```python
from build123d import *

# Parameters (mm, degrees)
ESQUISSE1_W                = 28.3
ESQUISSE1_H                = 28.3
ESQUISSE1_W_2              = 20.3
ESQUISSE1_H_2              = 20.3
ESQUISSE1_W_3              = 4
ESQUISSE1_H_3              = 2
BOSS_EXTRU_1_DEPTH         = 20
BOSS_EXTRU_7_DEPTH         = 20
ESQUISSE2_W                = 8.5
ESQUISSE2_H                = 20
ESQUISSE2_R                = 1.7
BOSS_EXTRU_2_DEPTH         = 2
ESQUISSE2_3_W              = 8.5
ESQUISSE2_3_H              = 20
BOSS_EXTRU_3_DEPTH         = 3
ESQUISSE3_W                = 8.5
ESQUISSE3_H                = 20
ESQUISSE3_R                = 1.7
BOSS_EXTRU_4_DEPTH         = 2
ESQUISSE5_W                = 8.5
ESQUISSE5_H                = 20
ESQUISSE5_R                = 3
BOSS_EXTRU_5_DEPTH         = 2
BOSS_EXTRU_6_DEPTH         = 20
BOSS_EXTRU_6_DEPTH_BACK    = 20
ESQUISSE6_W                = 28.3
ESQUISSE6_H                = 28.3
ESQUISSE6_W_2              = 15.3
ESQUISSE6_H_2              = 15.3
BOSS_EXTRU_12_REACH        = 59.663
ESQUISSE20_W               = 28.3
ESQUISSE20_H               = 28.3
ENL_V_MAT_EXTRU_1_REACH    = 81.469
ESQUISSE7_W                = 6.5
ESQUISSE7_H                = 2
ENL_V_MAT_EXTRU_2_REACH    = 82.765
ESQUISSE8_W                = 14.15
ESQUISSE8_H                = 2
ESQUISSE9_W                = 8.5
ESQUISSE9_H                = 40
BOSS_EXTRU_8_DEPTH         = 5
ESQUISSE9_4_R              = 1.7
BOSS_EXTRU_9_DEPTH         = 2
ESQUISSE10_W               = 8.5
ESQUISSE10_H               = 40
ESQUISSE10_R               = 1.7
BOSS_EXTRU_10_DEPTH        = 2
ESQUISSE11_W               = 8.5
ESQUISSE11_H               = 40
ESQUISSE11_R               = 3
BOSS_EXTRU_11_DEPTH        = 2
NERVURE4_REACH             = 81.469
ESQUISSE14_WALL_W          = 172.71321229
ESQUISSE14_WALL_H          = 5
NERVURE10_REACH            = 81.469
ESQUISSE16_WALL_W          = 173.426178518
ESQUISSE16_WALL_H          = 5
R_P_TITION_LIN_AIRE1_COUNT = 3
R_P_TITION_LIN_AIRE1_PITCH = 17.5
NERVURE11_REACH            = 93.316
ESQUISSE17_WALL_W          = 197.121376998
ESQUISSE17_WALL_H          = 5
NERVURE17_REACH            = 75.701
ESQUISSE19_WALL_W          = 161.177827304
ESQUISSE19_WALL_H          = 5
R_P_TITION_LIN_AIRE2_COUNT = 2
R_P_TITION_LIN_AIRE2_PITCH = 15
R_P_TITION_LIN_AIRE3_COUNT = 2
R_P_TITION_LIN_AIRE3_PITCH = 15
ENL_V_MAT_EXTRU_3_REACH    = 75.701
ESQUISSE21_W               = 4
ESQUISSE21_H               = 2.012776607


with BuildPart() as part:
    # Esquisse1 → Boss.-Extru.1 (new body)
    # profile 1 of 2: a face of its own
    with BuildSketch(Plane.XY):
        Rectangle(ESQUISSE1_W, ESQUISSE1_H)
        Rectangle(ESQUISSE1_W_2, ESQUISSE1_H_2, mode=Mode.SUBTRACT)
    # profile 2 of 2: a face of its own
    with BuildSketch(Plane.XY):
        with Locations((12.15, -1)):
            Rectangle(ESQUISSE1_W_3, ESQUISSE1_H_3)
    extrude(amount=BOSS_EXTRU_1_DEPTH)

    # Esquisse1<3> → Boss.-Extru.7 (add)
    with BuildSketch(Plane.XY):
        Polygon((14.15, 14.15), (-14.15, 14.15), (-14.15, -14.15), (14.15, -14.15), (14.15, -2), (10.15, -2), (10.15, -10.15), (-10.15, -10.15), (-10.15, 10.15), (10.15, 10.15), (10.15, 0), (14.15, 0), align=None)
    extrude(amount=-BOSS_EXTRU_7_DEPTH)

    # Esquisse2 → Boss.-Extru.2 (add)
    with BuildSketch(Plane(origin=(0, 2, 0), x_dir=(-1, 0, 0), z_dir=(0, -1, 0))):
        with Locations((-18.4, 10)):
            Rectangle(ESQUISSE2_W, ESQUISSE2_H)
        with Locations(Location((-18.4, 10, 0), (0, 0, 180))):
            Circle(ESQUISSE2_R, mode=Mode.SUBTRACT)
    extrude(amount=BOSS_EXTRU_2_DEPTH)

    # Esquisse2<3> → Boss.-Extru.3 (add)
    with BuildSketch(Plane(origin=(0, 2, 0), x_dir=(-1, 0, 0), z_dir=(0, -1, 0))):
        with Locations((-18.4, 10)):
            Rectangle(ESQUISSE2_3_W, ESQUISSE2_3_H)
        Polygon((-15.65, 11.58771324), (-15.65, 8.41228676), (-18.4, 6.824573519), (-21.15, 8.41228676), (-21.15, 11.58771324), (-18.4, 13.175426481), align=None, mode=Mode.SUBTRACT)
    extrude(amount=-BOSS_EXTRU_3_DEPTH)

    # Esquisse3 → Boss.-Extru.4 (add)
    with BuildSketch(Plane(origin=(0, -2, 0), x_dir=(1, 0, 0), z_dir=(0, 1, 0))):
        with Locations((18.4, 10)):
            Rectangle(ESQUISSE3_W, ESQUISSE3_H)
        with Locations((18.4, 10)):
            Circle(ESQUISSE3_R, mode=Mode.SUBTRACT)
    extrude(amount=-BOSS_EXTRU_4_DEPTH)

    # Esquisse5 → Boss.-Extru.5 (add)
    with BuildSketch(Plane.XZ.offset(4)):
        with Locations((18.4, -10)):
            Rectangle(ESQUISSE5_W, ESQUISSE5_H)
        with Locations((18.4, -10)):
            Circle(ESQUISSE5_R, mode=Mode.SUBTRACT)
    extrude(amount=BOSS_EXTRU_5_DEPTH)


with BuildPart() as body_2:
    # Esquisse6 → Boss.-Extru.6 (new, two sides: drawn at the far end of the back side and taken through both)
    with BuildSketch(Plane(origin=(0, -11.88296393, 7.558102729), x_dir=(-1, 0, 0), z_dir=(0, -0.8660254037844382, 0.5000000000000011)).offset(-BOSS_EXTRU_6_DEPTH_BACK)):
        with Locations((0, -37.941481073)):
            Rectangle(ESQUISSE6_W, ESQUISSE6_H)
        with Locations((0, -37.941481073)):
            Rectangle(ESQUISSE6_W_2, ESQUISSE6_H_2, mode=Mode.SUBTRACT)
    extrude(amount=BOSS_EXTRU_6_DEPTH + BOSS_EXTRU_6_DEPTH_BACK)

    # Esquisse20 → Boss.-Extru.12 (add, up to next)
    with BuildSketch(Plane.XY.offset(20), mode=Mode.PRIVATE) as boss_extru_12_sk1:
        Rectangle(ESQUISSE20_W, ESQUISSE20_H)
    boss_extru_12_tool1 = extrude(boss_extru_12_sk1.sketch, amount=BOSS_EXTRU_12_REACH, mode=Mode.PRIVATE) - body_2.part

    add(part.part)  # Boss.-Extru.12 merges part
    add(boss_extru_12_tool1.solids().sort_by_distance((0, 0, 20))[0])

    # Esquisse7 → Enlèv. mat.-Extru.1 (cut, up to next)
    with BuildSketch(Plane(origin=(0, -29.505485507, 17.035), x_dir=(1, 0, 0), z_dir=(0, -0.866025403784438, 0.5000000000000011)), mode=Mode.PRIVATE) as enl_v_mat_extru_1_sk1:
        with Locations((10.9, 39.545508076)):
            Rectangle(ESQUISSE7_W, ESQUISSE7_H)
    enl_v_mat_extru_1_tool1 = extrude(enl_v_mat_extru_1_sk1.sketch, amount=-ENL_V_MAT_EXTRU_1_REACH, mode=Mode.PRIVATE) & body_2.part
    add(enl_v_mat_extru_1_tool1.solids().sort_by_distance((10.9, -9.732731, 51.282415))[0], mode=Mode.SUBTRACT)

    # Esquisse8 → Enlèv. mat.-Extru.2 (cut, up to next)
    with BuildSketch(Plane.XZ.offset(14.15), mode=Mode.PRIVATE) as enl_v_mat_extru_2_sk1:
        with Locations((7.075, 9.169506309)):
            Rectangle(ESQUISSE8_W, ESQUISSE8_H)
    enl_v_mat_extru_2_tool1 = extrude(enl_v_mat_extru_2_sk1.sketch, amount=-ENL_V_MAT_EXTRU_2_REACH, mode=Mode.PRIVATE) & body_2.part
    add(enl_v_mat_extru_2_tool1.solids().sort_by_distance((7.075, -14.15, 9.169506))[0], mode=Mode.SUBTRACT)

    # Esquisse9 → Boss.-Extru.8 (add)
    with BuildSketch(Plane(origin=(0, 19.272754038, 33.381389195), x_dir=(1, 0, 0), z_dir=(0, 0.5000000000000011, 0.866025403784438))):
        with Locations((18.4, -14.07)):
            Rectangle(ESQUISSE9_W, ESQUISSE9_H)
        Polygon((18.4, -7.245426481), (21.15, -5.65771324), (21.15, -2.48228676), (18.4, -0.894573519), (15.65, -2.48228676), (15.65, -5.65771324), align=None, mode=Mode.SUBTRACT)
        Polygon((18.4, -20.894573519), (21.15, -22.48228676), (21.15, -25.65771324), (18.4, -27.245426481), (15.65, -25.65771324), (15.65, -22.48228676), align=None, mode=Mode.SUBTRACT)
    extrude(amount=-BOSS_EXTRU_8_DEPTH)

    # Esquisse9<4> → Boss.-Extru.9 (add)
    # profile 1 of 2: a face of its own
    with BuildSketch(Plane(origin=(0, 19.272754038, 33.381389195), x_dir=(1, 0, 0), z_dir=(0, 0.5000000000000011, 0.866025403784438))):
        Polygon((15.65, -5.65771324), (18.4, -7.245426481), (21.15, -5.65771324), (21.15, -2.48228676), (18.4, -0.894573519), (15.65, -2.48228676), align=None)
        with Locations(Location((18.4, -4.07, 0), (0, 0, 270))):
            Circle(ESQUISSE9_4_R, mode=Mode.SUBTRACT)
    # profile 2 of 2: a face of its own
    with BuildSketch(Plane(origin=(0, 19.272754038, 33.381389195), x_dir=(1, 0, 0), z_dir=(0, 0.5000000000000011, 0.866025403784438))):
        Polygon((21.15, -22.48228676), (21.15, -25.65771324), (18.4, -27.245426481), (15.65, -25.65771324), (15.65, -22.48228676), (18.4, -20.894573519), align=None)
        with Locations(Location((18.4, -24.07, 0), (0, 0, 270))):
            Circle(ESQUISSE9_4_R, mode=Mode.SUBTRACT)
    extrude(amount=-BOSS_EXTRU_9_DEPTH)

    # Esquisse10 → Boss.-Extru.10 (add)
    with BuildSketch(Plane(origin=(0, 20.272754038, 35.113440003), x_dir=(-1, 0, 0), z_dir=(0, -0.5000000000000011, -0.866025403784438))):
        with Locations((-18.4, -14.07)):
            Rectangle(ESQUISSE10_W, ESQUISSE10_H)
        with Locations(Location((-18.4, -24.07, 0), (0, 0, 270))):
            Circle(ESQUISSE10_R, mode=Mode.SUBTRACT)
        with Locations(Location((-18.4, -4.07, 0), (0, 0, 270))):
            Circle(ESQUISSE10_R, mode=Mode.SUBTRACT)
    extrude(amount=-BOSS_EXTRU_10_DEPTH)

    # Esquisse11 → Boss.-Extru.11 (add)
    with BuildSketch(Plane(origin=(0, 21.272754038, 36.84549081), x_dir=(1, 0, 0), z_dir=(0, 0.5000000000000011, 0.866025403784438))):
        with Locations((18.4, -14.07)):
            Rectangle(ESQUISSE11_W, ESQUISSE11_H)
        with Locations(Location((18.4, -4.07, 0), (0, 0, 270))):
            Circle(ESQUISSE11_R, mode=Mode.SUBTRACT)
        with Locations(Location((18.4, -24.07, 0), (0, 0, 270))):
            Circle(ESQUISSE11_R, mode=Mode.SUBTRACT)
    extrude(amount=BOSS_EXTRU_11_DEPTH)

    # Esquisse14 wall → Nervure4 (add, up to next)
    with BuildSketch(Plane(origin=(18.4, -5.195231469, 59.141595139), x_dir=(0.721811427089, -0.346044890046, -0.599367331272), z_dir=(0.692089780103, 0.360905713545, 0.625107032601)), mode=Mode.PRIVATE) as nervure4_sk1:
        with Locations((0, 2.5)):
            Rectangle(ESQUISSE14_WALL_W, ESQUISSE14_WALL_H)
    nervure4_tool1 = extrude(nervure4_sk1.sketch, amount=-NERVURE4_REACH, mode=Mode.PRIVATE) - body_2.part
    nervure4 = nervure4_tool1.solids().sort_by_distance((18.4, -5.195231469, 59.141595139))[0]
    add(nervure4)

    # Esquisse16 wall → Nervure10 (add, up to next)
    with BuildSketch(Plane(origin=(18.4, -15.020231469, 42.124195954), x_dir=(-0.680604645529, -0.366325441564, -0.634494276844), z_dir=(0.732650883085, -0.340302322764, -0.589420912962)), mode=Mode.PRIVATE) as nervure10_sk1:
        with Locations((0, 2.5)):
            Rectangle(ESQUISSE16_WALL_W, ESQUISSE16_WALL_H)
    nervure10_tool1 = extrude(nervure10_sk1.sketch, amount=-NERVURE10_REACH, mode=Mode.PRIVATE) - body_2.part
    nervure10 = nervure10_tool1.solids().sort_by_distance((18.4, -15.020231469, 42.124195954))[0]
    add(nervure10)

    # Répétition linéaire1: Nervure4, Nervure10 ×3
    with Locations(*[Vector(0, 0.8660254037844382, -0.500000000000001) * (i * R_P_TITION_LIN_AIRE1_PITCH) for i in range(1, R_P_TITION_LIN_AIRE1_COUNT)]):
        add(nervure4)
        add(nervure10)

    # Esquisse17 wall → Nervure11 (add, up to next)
    with BuildSketch(Plane(origin=(18.4, 9.575, -20), x_dir=(-0.680604645507, 0.732650883105, 0), z_dir=(0.732650883105, 0.680604645507, 0)), mode=Mode.PRIVATE) as nervure11_sk1:
        with Locations((0, 2.5)):
            Rectangle(ESQUISSE17_WALL_W, ESQUISSE17_WALL_H)
    nervure11_tool1 = extrude(nervure11_sk1.sketch, amount=-NERVURE11_REACH, mode=Mode.PRIVATE) - body_2.part
    nervure11 = nervure11_tool1.solids().sort_by_distance((18.4, 9.575, -20))[0]
    add(nervure11)

    # Esquisse19 wall → Nervure17 (add, up to next)
    with BuildSketch(Plane(origin=(18.4, -10.075, 0), x_dir=(-0.721811427095, -0.692089780097, 0), z_dir=(0.692089780097, -0.721811427095, 0)), mode=Mode.PRIVATE) as nervure17_sk1:
        with Locations((0, 2.5)):
            Rectangle(ESQUISSE19_WALL_W, ESQUISSE19_WALL_H)
    nervure17_tool1 = extrude(nervure17_sk1.sketch, amount=-NERVURE17_REACH, mode=Mode.PRIVATE) - body_2.part
    nervure17 = nervure17_tool1.solids().sort_by_distance((18.4, -10.075, 0))[0]
    add(nervure17)

    # Répétition linéaire2: Nervure17 ×2
    with Locations(*[(0, 0, -i * R_P_TITION_LIN_AIRE2_PITCH) for i in range(1, R_P_TITION_LIN_AIRE2_COUNT)]):
        add(nervure17)

    # Répétition linéaire3: Nervure11 ×2
    with Locations(*[(0, 0, i * R_P_TITION_LIN_AIRE3_PITCH) for i in range(1, R_P_TITION_LIN_AIRE3_COUNT)]):
        add(nervure11)

    # Esquisse21 → Enlèv. mat.-Extru.3 (cut, up to next)
    with BuildSketch(Plane(origin=(0, 0, 0), x_dir=(-1, 0, 0), z_dir=(0, 0, -1)), mode=Mode.PRIVATE) as enl_v_mat_extru_3_sk1:
        with Locations((-12.15, -0.993611697)):
            Rectangle(ESQUISSE21_W, ESQUISSE21_H)
    enl_v_mat_extru_3_tool1 = extrude(enl_v_mat_extru_3_sk1.sketch, amount=-ENL_V_MAT_EXTRU_3_REACH, mode=Mode.PRIVATE) & body_2.part
    add(enl_v_mat_extru_3_tool1.solids().sort_by_distance((12.15, -0.993612, 0))[0], mode=Mode.SUBTRACT)


solid = body_2.part
```
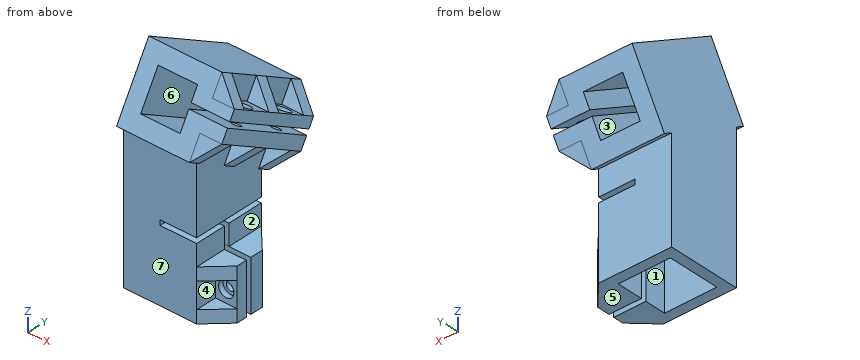
Work out the finished part from the listing and answer in its coordinate system (mm). Face numbers are marked on the shaded views. A direction names the side the tool comes from. Coordinates: 2 decimals unless noted, no trailing zeros. Loops run counter-clockwise (first coordinate to the right, second up) from the corner with the lowest first, then second, coordinate; pieces in that order, holes last. Notation, with made-up numbers: (11, 89.25) - (27, 89.25) arc R23 ccw to (27, 128.25) - close; hole circle Ø5 at (28, 22.5). An arc over 180 degrees is marked (long way). Use a Markdown table: item, result.
Item 1: Given pin 1 Ø1 at (y, z) = (-11.5, 9.5) entering from +X; pin 2 Ø12 at (x, z) = (-7, 53.5) entering from +Y; pin 3 Ø8 at (x, y) = (2.5, 23) entering from -Z; pin 4 Ø7 at (x, y) = (19.5, 11.5) entering from -Z, each flat-ended and moving along its own axis, determine where each tip first touches the part or whether it passes through.
Evaluation:
| item | result |
|---|---|
| pin 1 | stops at x = 0 |
| pin 2 | stops at y = 23.12 |
| pin 3 | stops at z = 21.05 |
| pin 4 | stops at z = -20 |
Item 2: Find section B-B, the plane z = -10. State how many separate pieces and enclosed holes the cut face has, and give its area (3 significant figures).
Evaluation:
| item | result |
|---|---|
| separate pieces | 3 |
| enclosed holes | 0 |
| area | 415 mm2 |
Item 3: For the marked faces 1, 2, 3 and 4, determine the directions among +Z, -Z, +X, -X, +Y, -Y from which every point of the face is accessible in a straight line to the end or side of a thin tool.
Evaluation:
| item | result |
|---|---|
| face 1 | -Z |
| face 2 | +X, +Y, -Y |
| face 3 | none |
| face 4 | +X, -Y |
Item 4: Find section C-C, the plane x = -1. Determine the outline of the cut face in (y, z).
Evaluation:
| item | result |
|---|---|
| outline | (-17.31, 38.16) - (-14.15, 36.34) - (-14.15, -20) - (-10.15, -20) - (-10.15, 20) - (10.15, 20) - (10.15, -20) - (14.15, -20) - (14.15, 20) - (17.33, 18.16) - (20.58, 23.79) - (-14.06, 43.79) - close; (-6.41, 57.04) - (28.23, 37.04) - (31.48, 42.67) - (-3.16, 62.67) - close |
Item 5: Find section A-A, the plane x = 6. Determine the outline of the cut face in (y, z).
Evaluation:
| item | result |
|---|---|
| outline | (-17.31, 38.16) - (-14.15, 36.34) - (-14.15, 10.17) - (-10.15, 10.17) - (-10.15, 20) - (10.15, 20) - (10.15, 10.17) - (14.15, 10.17) - (14.15, 20) - (17.33, 18.16) - (20.58, 23.79) - (-14.06, 43.79) - close; (-14.15, -20) - (-10.15, -20) - (-10.15, 8.17) - (-14.15, 8.17) - close; (-6.41, 57.04) - (28.23, 37.04) - (31.48, 42.67) - (-3.16, 62.67) - close; (10.15, -20) - (14.15, -20) - (14.15, 8.17) - (10.15, 8.17) - close |
Item 6: Consider probe 1 along Y at (x, z) = (15.5, -8); probe 2 along Y at (x, z) = (6, -16); probe 3 along X at (y, z) = (14, 42.5). Determine where each line is inside the solid, lowest interval first. Write a range as from..to.
Evaluation:
| item | result |
|---|---|
| probe 1 | y = -6..-2, 0..5 |
| probe 2 | y = -14.15..-10.15, 10.15..14.15 |
| probe 3 | x = -14.15..-7.65, 7.65..22.65 |
Item 7: The mould has two halves that part along Z. Classify the marked faces 5, 6 and 7: +Z half, -Z half, draft (parallel to the pull), parting line (faces both ways), or undercut.
Evaluation:
| item | result |
|---|---|
| face 5 | -Z half |
| face 6 | undercut |
| face 7 | draft |
